For this review, take the finished solid that the model builds, in its own axes (mm). A direction names the side the tool comes from. Coordinates: 2 decimals unless noted, no trailing zeros. Loops run counter-clockwise (first coordinate to the right, second up) from the corner with the lowest first, then second, coordinate; pieces in that order, holes last. Notation, with made-up numbers: (85.25, 50.25) -> (137.25, 50.25) arc R30 ccw to (137.25, 82.25) -> close; hole circle Ø11 at (77.5, 0). An arc over 180 degrees is marked (long way). Answer in a Markdown table with one row per item.
from build123d import *

# Parameters (mm, degrees)
SKETCH_1_W      = 2
SKETCH_1_H      = 15
EXTRUDE_1_DEPTH = 2
REVOLVE_1_ANGLE = 180


with BuildPart() as part:
    # Эскиз1 → Бобышка-Вытянуть1 (new body)
    with BuildSketch(Plane(origin=(0, 0, 0), x_dir=(1, 0, 0), z_dir=(0, 1, 0))):
        with Locations((0, 7.5)):
            Rectangle(SKETCH_1_W, SKETCH_1_H)
    extrude(amount=EXTRUDE_1_DEPTH)

    # Эскиз2 → Повернуть1 (revolve)
    with BuildSketch(Plane(origin=(0, 0, 0), x_dir=(1, 0, 0), z_dir=(0, 1, 0))):
        with BuildLine():
            Line((0, 0.8), (0, 0))
            ThreePointArc((0, 0), (-15, -15), (0, -30))
            Line((0, -30), (0, -30.8))
            ThreePointArc((0, -30.8), (-15.8, -15), (0, 0.8))
        make_face()
    revolve(axis=Axis((0, 0, 15), (0, 0, -1)), revolution_arc=REVOLVE_1_ANGLE)


solid = part.part
Item 1: Take a section at A-A, the plane z = -9.5. State the section outline as (x, y) points.
Worked answers:
| item | result |
|---|---|
| outline | (-1, 0) -> (1, 0) -> (1, 2) -> (-1, 2) -> close |
Item 2: Take a section at C-C, the plane x = 4. State the section outline as (y, z) points, and give its area (3 significant figures).
Worked answers:
| item | result |
|---|---|
| outline | (0, -0.29) arc R15.29 ccw to (0, 30.29) -> (0, 29.46) arc R14.46 cw to (0, 0.54) -> close |
| area | 38.7 mm² |
Item 3: Take a section at D-D, the plane y = 12.5. State the section outline as (x, z) points.
Worked answers:
| item | result |
|---|---|
| outline | circle Ø19.33 at (0, 15); hole circle Ø16.58 at (0, 15) |
Item 4: Insertion check: pin 1 (10 mm diameter, centred on x = -5.5, z = 22.5, fed in from +Y); pin 2 (8 mm diameter, centred on y = 1.5, z = 21, fed in from +X); pin 3 (0.6 mm diameter, centred on x = 0, z = -6, fed in from +Y); pin 4 (8 mm diameter, centred on y = 1.5, z = 16.5, fed in from +X). Each pin has a flat end and moves straight along its axis. Give the tip position at first contact, or say it passes through.
Worked answers:
| item | result |
|---|---|
| pin 1 | y = 15.2 |
| pin 2 | x = 15.65 |
| pin 3 | y = 2 |
| pin 4 | x = 15.8 |
Item 5: For faces 1 (the flat face through (0, 1, -15)), 2 (the flat face through (-1, 1, -8)), 3 (the flat face through (-6, 0, 1)), 4 (the flat face through (1, 1, -8)), 5 (the flat face through (0, 2, -8)), list the 3-axis set-ups (+Z, -Z, +X, -X, +Y, -Y) from which the entire face can be reached by the end or side of a thin tool; tool diameter is ignored.
Worked answers:
| item | result |
|---|---|
| face 1 | -Z, +X, -X, +Y, -Y |
| face 2 | -Z, -X, +Y, -Y |
| face 3 | +Z, -Z, +X, -X, -Y |
| face 4 | -Z, +X, +Y, -Y |
| face 5 | -Z, +X, -X, +Y |
Item 6: For L1, parallel to Z at x = -10.5, y = 3.5; L2, parallel to X at y = 11, z = 13; L3, parallel to Z at x = -11, y = 3.5, list the stretches that pass through material, from the lowest coordinate up.
Worked answers:
| item | result |
|---|---|
| L1 | 3.72 to 4.88, 25.12 to 26.28 |
| L2 | -11.16 to -10, 10 to 11.16 |
| L3 | 4.21 to 5.42, 24.58 to 25.79 |
Item 7: Take a section at B-B, the plane y = 1.5. State the section outline as (x, z) points, and give its area (3 significant figures).
Worked answers:
| item | result |
|---|---|
| outline | (-1, -15) -> (1, -15) -> (1, -0.7) arc R15.73 ccw (long way) to (-1, -0.7) -> close; hole circle Ø29.85 at (0, 15) |
| area | 106 mm² |
